Model file for the job. Use its own axes, mm. A direction names the side the tool comes from. Coordinates: 2 decimals unless noted, no trailing zeros. Order: outer loops, then holes, each group sorted by start corner. A loop starts at its lowest first (then second) coordinate and runs counter-clockwise, first axis right, second up. Notation, with made-up numbers: (74.25, 17) -> (130.25, 17) arc R6 cw to (130.25, 27) -> close; hole circle Ø5 at (82.5, -34.75). An arc over 180 degrees is marked (long way). Return JSON: item names as keys, results as strings. Group by question number.
1) Which spindle directions (+Z, -Z, +X, -X, +Y, -Y) get a long thin tool onto all of the face, cutting with end or side? Do faces 1 (the cylindrical face through (381.53, -120.15, -4.83)), 2 (the flat face through (-6, 6, -344.901)). Say none if no direction does.
2) Probe line 1 (Z direction, x = -227.5, y = 196.5); line 2 (X direction, y = -7, z = -25.5); line 3 (X direction, y = -328, z = 411.5). List the from-to ranges inside material, lowest first.
3) Flat gauge pins, fed straight in: pin 1 (1.5 mm diameter, centred on x = -51.5, z = 372.5, fed in from -Y); pin 2 (10 mm diameter, centred on y = -118.5, z = 196, fed in from -X); pin 3 (1 mm diameter, centred on x = 284.5, z = 335.5, fed in from -Y). Where does each tip first touch, or does it go through?
4) Cut at D-D (z = 421). Write the cut outline in (x, y), and give its area (3 significant figures).
5) Cut at C-C (z = -284). Write the cut outline in (x, y), and give its area (3 significant figures).
Autodesk Inventor part; units mm, degrees
ref_plane "YZ Plane" through (0, 0, 0) normal (1, 0, 0) x (0, 1, 0)
ref_plane "XZ Plane" through (0, 0, 0) normal (0, 1, 0) x (-1, 0, 0)
ref_plane "XY Plane" through (0, 0, 0) normal (0, 0, 1) x (1, 0, 0)
sketch "Sketch1" plane through (0, 0, 0) normal (0, 0, 1) x (1, 0, 0)
  circle A0 centre (0, 0) radius 400
  dimension "d0" = 800
extrude "Extrusion1" add sketch "Sketch1" along normal mid plane 689.802
sketch "Sketch2" plane through (0, 0, 344.901) normal (0, 0, 1) x (1, 0, 0)
  circle A0 centre (0, 0) radius 500
  dimension "d3" = 1000
extrude "Extrusion2" add sketch "Sketch2" along normal blind 200
fillet "Fillet1" radius 200 1 edges at (-500, 0, 544.901)
properties part number "06_LastArmChop"
Answers below:
{
 "1": {"face 1": "-Z", "face 2": "-Z, +X, -X, +Y, -Y"},
 "2": {"line 1": "z = -344.9 to 544.9", "line 2": "x = -399.94 to 399.94", "line 3": "x = -362.12 to 362.12"},
 "3": {"pin 1": "stops at y = -495.55", "pin 2": "stops at x = -383.56", "pin 3": "stops at y = -281.68"},
 "4": {"outline": "circle Ø969.91 at (0, 0)", "area": "739,000 mm^2"},
 "5": {"outline": "circle Ø800 at (0, 0)", "area": "503,000 mm^2"}
}
